from build123d import *

# Parameters (mm, degrees)
F0_W          = 100
F0_H          = 35
F1_DEPTH      = 30
F2_W          = 5
F2_H          = 20
F2_W_2        = 30
F2_H_2        = 5
F3_DEPTH      = 100
F5_DEPTH      = 100
F5_DEPTH_BACK = 74.2
F7_DEPTH      = 100
F7_DEPTH_BACK = 100.7


with BuildPart() as f1:
    # F0 (on Right) → F1 (new body, symmetric)
    with BuildSketch(Plane.YZ):
        Rectangle(F0_W, F0_H)
    extrude(amount=F1_DEPTH, both=True)

    # F2 (on face) → F3 (cut)
    with BuildSketch(Plane.XZ.offset(50)):
        with Locations((-27.5, -7.5)):
            Rectangle(F2_W, F2_H)
        with Locations((0, -15)):
            Rectangle(F2_W_2, F2_H_2)
        with Locations((27.5, -7.5)):
            Rectangle(F2_W, F2_H)
    extrude(amount=-F3_DEPTH, mode=Mode.SUBTRACT)

    # F4 (on Front) → F5 (cut, two sides)
    with BuildSketch(Plane.XZ) as f5_sk:
        Polygon((30.0000030547, 11.5), (30.0000030547, 17.5), (24, 17.5), align=None)
        Polygon((-30.0000030547, 11.5), (-24, 17.5), (-30.0000030547, 17.5), align=None)
    extrude(amount=-F5_DEPTH, mode=Mode.SUBTRACT)
    extrude(f5_sk.sketch, amount=F5_DEPTH_BACK, mode=Mode.SUBTRACT)

    # F6 (on Front) → F7 (cut, two sides)
    with BuildSketch(Plane.XZ) as f7_sk:
        Polygon((2.5, -5.5), (2.5, -1.5), (21.5, 17.5), (-21.5, 17.5), (-2.5, -1.5), (-2.5, -5.5), align=None)
    extrude(amount=-F7_DEPTH, mode=Mode.SUBTRACT)
    extrude(f7_sk.sketch, amount=F7_DEPTH_BACK, mode=Mode.SUBTRACT)


solid = f1.part
Check sheet for the modelled part. Datum: model origin and axes. Units: mm. A direction names the side the tool comes from. Coordinates: 2 decimals unless noted, no trailing zeros. Write each loop counter-clockwise with the first axis right and the second up, starting at its lowest first coordinate (ties: lowest second). Pieces come first, ordered by that corner, then holes.
Item 1: Depth check by flat-ended pin: pin 1 Ø10 at (x, y) = (-14.5, -19.5) entering from +Z; pin 2 Ø1.5 at (x, y) = (27, 12.5) entering from -Z; pin 3 Ø10 at (y, z) = (-22.5, -3.5) entering from -X. Enter the tip coordinate at first touch or a pass-through.
Numbers:
pin 1: stops at z = 15.5
pin 2: stops at z = 2.5
pin 3: stops at x = -25
Item 2: Mould release check, pull along X, two halves, no side actions. Record for faces 1 (the face through (-12, 1, 8)), 2 (the face through (27, 0.7, 14.5)), 3 (the face through (-28, -1, 2.5)): released by +X, released by -X, zero draft, split by the parting line, or undercut.
Numbers:
face 1: undercut
face 2: released by +X
face 3: zero draft
Item 3: Cross-section at A-A on z = 0. Record the boundary of the cut face in (x, y).
Numbers:
outline: (-25, -50) - (-4, -50) - (-4, 50) - (-25, 50) - close; (4, -50) - (25, -50) - (25, 50) - (4, 50) - close
Item 4: Cross-section at D-D on z = -10. Record the boundary of the cut face in (x, y), then the cut area to 3 significant figures.
Numbers:
outline: (-25, -50) - (25, -50) - (25, 50) - (-25, 50) - close
area: 5,000 mm2
Item 5: Access from +Z, -Z, +X, -X, +Y, -Y to the whole of each face (thin tool, end or side, straight path). Record for faces 4 (the face through (15, -1, -15)), 5 (the face through (-2.5, 1, -3)), 6 (the face through (27, -1, 2.5)).
Numbers:
face 4: -Z, +Y, -Y
face 5: +Z, +Y, -Y
face 6: -Z, +X, +Y, -Y
Item 6: Cross-section at B-B on y = 12. Record the boundary of the cut face in (x, z), then the cut area to 3 significant figures.
Numbers:
outline: (-30, 2.5) - (-25, 2.5) - (-25, -17.5) - (-15, -17.5) - (-15, -12.5) - (15, -12.5) - (15, -17.5) - (25, -17.5) - (25, 2.5) - (30, 2.5) - (30, 11.5) - (24, 17.5) - (21.5, 17.5) - (2.5, -1.5) - (2.5, -5.5) - (-2.5, -5.5) - (-2.5, -1.5) - (-21.5, 17.5) - (-24, 17.5) - (-30, 11.5) - close
area: 1,240 mm2
Item 7: Cross-section at C-C on x = -13.5. Record the boundary of the cut face in (y, z), then the cut area to 3 significant figures.
Numbers:
outline: (-50, -12.5) - (50, -12.5) - (50, 9.5) - (-50, 9.5) - close
area: 2,200 mm2
Item 8: Scan lines: probe 1 along X at (y, z) = (37, -3); probe 2 along X at (y, z) = (3, 11); probe 3 along Z at (x, y) = (19, 16.5). Record each from-to range of solid material in increasing order.
Numbers:
probe 1: x = -25 to -2.5, 2.5 to 25
probe 2: x = -30 to -15, 15 to 30
probe 3: z = -17.5 to 15
